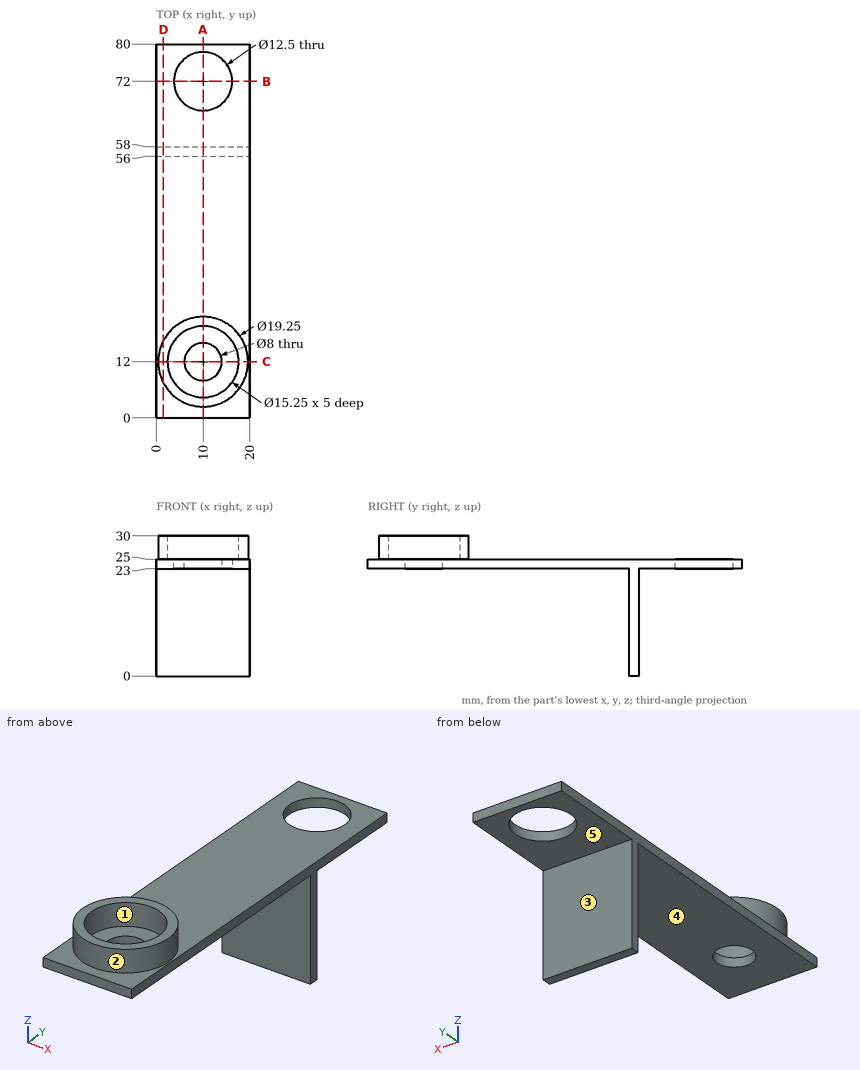
Can you work these out from the drawing? Everything is in mm from the part's minimum corner. A direction names the side the tool comes from. Round coordinates to 2 decimals unless told otherwise and drop trailing zeros. Write each loop counter-clockwise with the first axis right and the second up, starting at its lowest first coordinate (ties: lowest second). Pieces come first, ordered by that corner, then holes. Notation, with made-up numbers: (53.5, 62) - (64.5, 62) arc R12 ccw to (64.5, 73) - close; hole circle Ø10 at (33, 52). An arc over 180 degrees is marked (long way). Put each result on its own line as item: value. Start each with the question number.
(1) Will these pins go through, and if not, where does the flat tip stop? pin 1 (3 mm diameter, centred on x = 6.5, z = 25.5, fed in from -Y); pin 2 (1.5 mm diameter, centred on x = 8, y = 53, fed in from +Z); pin 3 (3 mm diameter, centred on x = 4, y = 51.5, fed in from -Z); pin 4 (12 mm diameter, centred on x = 6, z = 9.5, fed in from +Y).
(2) I want a section at D-D, the plane x = 1.5. Please give me the cut outline in (y, z), plus the area to 3 significant figures.
(3) I need wall thicknesses on probe 1 along Y at (x, z) = (10, 23.7); probe 2 along Y at (x, z) = (1.25, 20.5); probe 3 along Z at (x, y) = (18.5, 33). Which ranges of each line are inside material? Lowest first, please.
(4) I want a section at C-C, the plane y = 12. Please give me the cut outline in (x, z) (3 decimals), plus the area to 3 significant figures.
(5) I want a section at A-A, the plane x = 10. Please give me the cut outline in (y, z) (3 decimals).
(6) I want a section at B-B, the plane y = 72. Please give me the cut outline in (x, z).
(7) For the marked faces 4 and 5, which set-ups out of +Z, -Z, +X, -X, +Y, -Y let a thin tool reach every point of the face, with its end or its side?
(8) Thinking about a two-plate mould opening in X: for the marked faces 1, 2 and 3, which applies, released by +X, released by -X, zero draft, split by the parting line, or undercut?
Here are the results:
1. pin 1: stops at y = 0
1. pin 2: stops at z = 25
1. pin 3: stops at z = 23
1. pin 4: stops at y = 58
2. outline: (0, 23) - (56, 23) - (56, 0) - (58, 0) - (58, 23) - (80, 23) - (80, 25) - (16.52, 25) - (16.52, 30) - (7.48, 30) - (7.48, 25) - (0, 25) - close
2. area: 251 mm^2
3. probe 1: y = 0 to 8, 16 to 65.75, 78.25 to 80
3. probe 2: y = 56 to 58
3. probe 3: z = 23 to 25
4. outline: (0, 23) - (6, 23) - (6, 25) - (2.375, 25) - (2.375, 30) - (0.375, 30) - (0.375, 25) - (0, 25) - close; (14, 23) - (20, 23) - (20, 25) - (19.625, 25) - (19.625, 30) - (17.625, 30) - (17.625, 25) - (14, 25) - close
4. area: 44.0 mm^2
5. outline: (0, 23) - (8, 23) - (8, 25) - (4.375, 25) - (4.375, 30) - (2.375, 30) - (2.375, 25) - (0, 25) - close; (16, 23) - (56, 23) - (56, 0) - (58, 0) - (58, 23) - (65.75, 23) - (65.75, 25) - (21.625, 25) - (21.625, 30) - (19.625, 30) - (19.625, 25) - (16, 25) - close; (78.25, 23) - (80, 23) - (80, 25) - (78.25, 25) - close
6. outline: (0, 23) - (3.75, 23) - (3.75, 25) - (0, 25) - close; (16.25, 23) - (20, 23) - (20, 25) - (16.25, 25) - close
7. face 4: -Z, +X, -X, -Y
7. face 5: -Z, +X, -X, +Y
8. face 1: undercut
8. face 2: split by the parting line
8. face 3: zero draft
